The figure shows three views and two pictorial views of one solid part (mm, origin at its lowest corner). Answer the questions. A direction names the side the tool comes from. Round coordinates to 2 decimals unless told otherwise and drop trailing zeros. Loops run counter-clockwise (first coordinate to the right, second up) from the corner with the lowest first, then second, coordinate; pieces in that order, holes last. Notation, with made-up numbers: (58.25, -23) -> (89.25, -23) arc R12 cw to (89.25, 0) -> close; hole circle Ø10 at (62, -32.5). An arc over 180 degrees is marked (long way). Put each result on its own line as item: value.
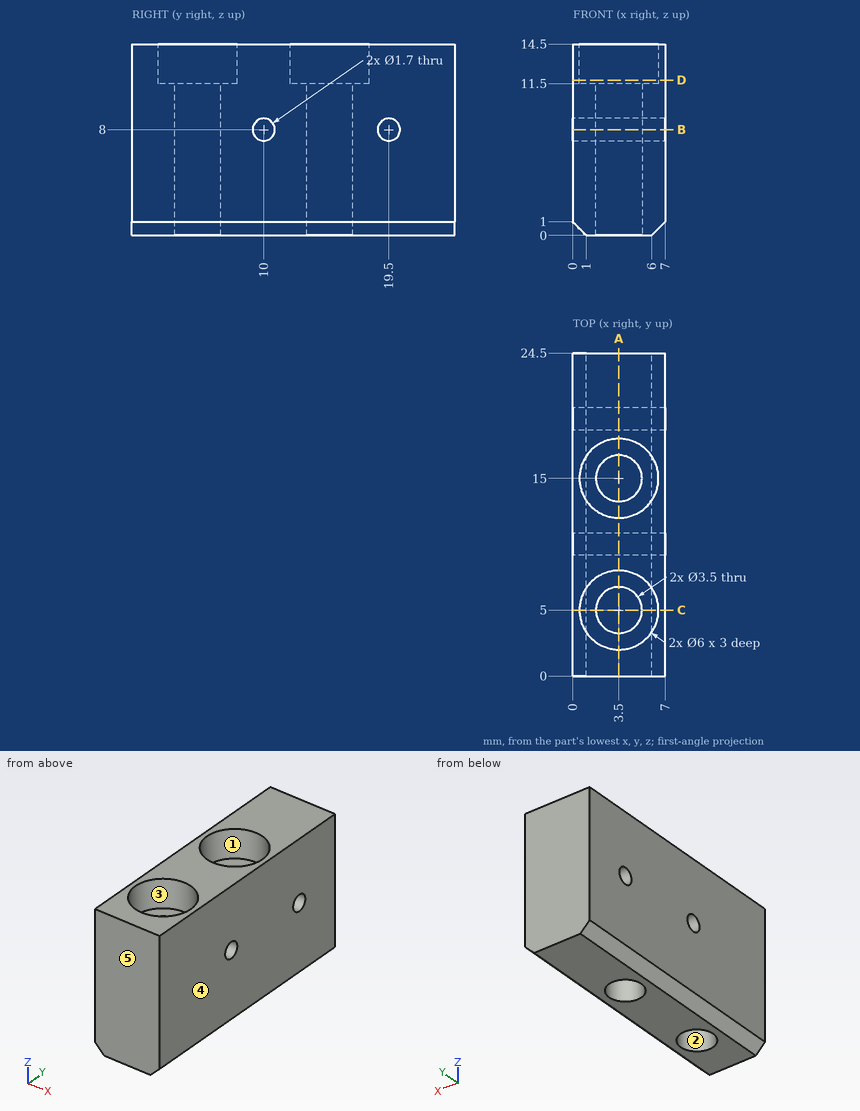
Item 1: The part is cut by section B-B (z = 8). Determine the outline of the cut face in (x, y).
Derived:
outline: (0, 0) -> (7, 0) -> (7, 9.15) -> (0, 9.15) -> close; (0, 10.85) -> (7, 10.85) -> (7, 18.65) -> (0, 18.65) -> close; (0, 20.35) -> (7, 20.35) -> (7, 24.5) -> (0, 24.5) -> close; hole circle Ø3.5 at (3.5, 5); hole circle Ø3.5 at (3.5, 15)
Item 2: The part is cut by section C-C (y = 5). Determine the outline of the cut face in (x, z), then the cut area to 4 significant figures.
Derived:
outline: (0, 1) -> (1, 0) -> (1.75, 0) -> (1.75, 11.5) -> (0.5, 11.5) -> (0.5, 14.5) -> (0, 14.5) -> close; (5.25, 0) -> (6, 0) -> (7, 1) -> (7, 14.5) -> (6.5, 14.5) -> (6.5, 11.5) -> (5.25, 11.5) -> close
area: 42.25 mm^2
Item 3: The part is cut by section A-A (x = 3.5). Determine the outline of the cut face in (y, z).
Derived:
outline: (0, 0) -> (3.25, 0) -> (3.25, 11.5) -> (2, 11.5) -> (2, 14.5) -> (0, 14.5) -> close; (6.75, 0) -> (13.25, 0) -> (13.25, 11.5) -> (12, 11.5) -> (12, 14.5) -> (8, 14.5) -> (8, 11.5) -> (6.75, 11.5) -> close; (16.75, 0) -> (24.5, 0) -> (24.5, 14.5) -> (18, 14.5) -> (18, 11.5) -> (16.75, 11.5) -> close; hole circle Ø1.7 at (10, 8); hole circle Ø1.7 at (19.5, 8)
Item 4: For a pull along Y with two mould halves and no side action, classify the marked faces 3, 4 and 5 as pulls with the +Y half, pulls with the -Y half, needs draft (parallel to the pull), parting line crosses it, or undercut.
Derived:
face 3: undercut
face 4: needs draft
face 5: pulls with the -Y half
Item 5: Which of the six approach directions +Z, -Z, +X, -X, +Y, -Y give full straight-line access (tool end or side, diameter ignored) to the marked faces 1 and 2?
Derived:
face 1: +Z
face 2: +Z, -Z
Item 6: The part is cut by section D-D (z = 11.75). Determine the outline of the cut face in (x, y), then the cut area to 3 significant figures.
Derived:
outline: (0, 0) -> (7, 0) -> (7, 24.5) -> (0, 24.5) -> close; hole circle Ø6 at (3.5, 5); hole circle Ø6 at (3.5, 15)
area: 115 mm^2
Item 7: Find the intervals of material crossed by line 1 along Y through (x, z) = (3.5, 12.35); line 2 along Y through (x, z) = (3.5, 9); line 3 along Y through (x, z) = (4, 7.25), in increasing order.
Derived:
line 1: y = 0 to 2, 8 to 12, 18 to 24.5
line 2: y = 0 to 3.25, 6.75 to 13.25, 16.75 to 24.5
line 3: y = 0 to 3.32, 6.68 to 9.6, 10.4 to 13.32, 16.68 to 19.1, 19.9 to 24.5
Item 8: Flat-ended cylindrical pins translate along their axes: pin 1 Ø1 at (y, z) = (19.5, 8) entering from +X; pin 2 Ø1.8 at (x, y) = (4.5, 14) entering from +Z. Find the tip coordinate at first contact, or state that the pin passes through.
Derived:
pin 1: passes through
pin 2: stops at z = 11.5
